CAD build for the part. Positions are in the model's coordinates, mm. A direction names the side the tool comes from. Round coordinates to 2 decimals unless told otherwise and drop trailing zeros. Order: outer loops, then holes, each group sorted by start corner. A loop starts at its lowest first (then second) coordinate and runs counter-clockwise, first axis right, second up. Notation, with made-up numbers: (-35.75, 65.5) -> (20.25, 65.5) arc R11 ccw to (20.25, 77.5) -> close; hole circle Ø5 at (-2.5, 89). An arc over 180 degrees is marked (long way). Answer as CSV lines item,"result". Start each with the question number.
from build123d import *
from build123d.topology import SkipClean

# Parameters (mm, degrees)
SKETCH1_R           = 4
SKETCH1_R_2         = 5.5
BOSS_EXTRUDE1_DEPTH = 2.5
BOSS_EXTRUDE2_START = -5
SKETCH2_R           = 4
BOSS_EXTRUDE2_DEPTH = 5
SKETCH3_R           = 2.25
CUT_EXTRUDE1_DEPTH  = 38.003378224
CUT_EXTRUDE2_DEPTH  = 6
CHAMFER1_SIZE       = 2
FILLET1_R           = 5
BOSS_EXTRUDE3_DEPTH = 10


# Read off the part's stored shape, not the designer's step: Boss-Extrude3
with BuildPart() as part:
    # Sketch1 → Boss-Extrude1 (new, symmetric)
    with BuildSketch(Plane(origin=(0, 0, 0), x_dir=(0, 0, -1), z_dir=(1, 0, 0))):
        with BuildLine():
            Line((-3.149551455, -9.491065569), (15.007926117, -15.51651229))
            ThreePointArc((15.007926117, -15.51651229), (20.188852348, -15.744399678), (24.717514421, -13.217514421))
            Line((24.717514421, -13.217514421), (27.121320344, -10.813708499))
            ThreePointArc((27.121320344, -10.813708499), (27.771638598, -9.840438453), (28, -8.692388155))
            Line((28, -8.692388155), (28, 23))
            Line((28, 23), (18, 23))
            Line((18, 23), (18, 13))
            ThreePointArc((18, 13), (17.121320344, 10.878679656), (15, 10))
            Line((15, 10), (0, 10))
            ThreePointArc((0, 10), (-9.871946507, 1.595202857), (-3.149551455, -9.491065569))
        make_face()
        Circle(SKETCH1_R, mode=Mode.SUBTRACT)
        with Locations((18, -6.5)):
            Circle(SKETCH1_R_2, mode=Mode.SUBTRACT)
    extrude(amount=BOSS_EXTRUDE1_DEPTH, both=True)

    # Sketch2 → Boss-Extrude2 (add)
    with SkipClean():  # the faces are left unmerged after this step: merging them gives an invalid solid
        with BuildSketch(Plane.ZY.offset(-2.5).offset(BOSS_EXTRUDE2_START)):
            with BuildLine():
                Line((0, 10), (-15, 10))
                ThreePointArc((-15, 10), (-17.121320344, 10.878679656), (-18, 13))
                Line((-18, 13), (-18, 23))
                Line((-18, 23), (-28, 23))
                Line((-28, 23), (-28, 9))
                ThreePointArc((-28, 9), (-27.414213562, 7.585786438), (-26, 7))
                Line((-26, 7), (-10.908712115, 7))
                ThreePointArc((-10.908712115, 7), (-9.225461292, 6.08012345), (-9.090593429, 4.166666667))
                ThreePointArc((-9.090593429, 4.166666667), (-9.651431629, 2.617225154), (-9.950203687, 0.996717904))
                ThreePointArc((-9.950203687, 0.996717904), (-7.653907103, -2.763910898), (-7.017714401, -7.124021658))
                ThreePointArc((-7.017714401, -7.124021658), (9.253113438, -3.792082767), (0, 10))
            make_face()
            Circle(SKETCH2_R, mode=Mode.SUBTRACT)
        extrude(amount=BOSS_EXTRUDE2_DEPTH)

    # Sketch3 → Cut-Extrude1 (cut, through all)
    with SkipClean():  # the faces are left unmerged after this step: merging them gives an invalid solid
        with BuildSketch(Plane.XY.offset(-18)):
            with Locations((2.5, 17)):
                Circle(SKETCH3_R)
        extrude(amount=-CUT_EXTRUDE1_DEPTH, mode=Mode.SUBTRACT)

    # Sketch4 → Cut-Extrude2 (cut)
    with SkipClean():  # the faces are left unmerged after this step: merging them gives an invalid solid
        with BuildSketch(Plane(origin=(0, 0, -28), x_dir=(-1, 0, 0), z_dir=(0, 0, -1))):
            Polygon((-6.05, 14.950406544), (-2.5, 12.900813089), (1.05, 14.950406544), (1.05, 19.049593456), (-2.5, 21.099186911), (-6.05, 19.049593456), align=None)
        extrude(amount=-CUT_EXTRUDE2_DEPTH, mode=Mode.SUBTRACT)

    # Chamfer1
    chamfer1_edges = [part.edges().sort_by_distance(p)[0] for p in [
        (-2.5, 23, -23),
        (7.5, 23, -23),
    ]]
    chamfer(chamfer1_edges, length=CHAMFER1_SIZE)

    # Fillet1
    fillet1_edges = [part.edges().sort_by_distance(p)[0] for p in [
        (5, -7.124021658, -7.017714401),
        (5, 0.996717904, -9.950203687),
    ]]
    fillet(fillet1_edges, radius=FILLET1_R)

    # Boss-Extrude3 outline → Boss-Extrude3 (add)
    with SkipClean():  # the faces are left unmerged after this step: merging them gives an invalid solid
        with BuildSketch(Plane(origin=(7.5, 0, 0), x_dir=(0, 0, -1), z_dir=(1, 0, 0))):
            with BuildLine():
                ThreePointArc((-2.463364838, -9.691843668), (0.945667306, -9.955185249), (4.244142914, -9.054681161))
                ThreePointArc((4.244142914, -9.054681161), (6.167964396, -7.465154449), (7.083924127, -5.143796649))
                ThreePointArc((7.083924127, -5.143796649), (7.6539625, -2.763757496), (8.736132305, -0.568663276))
                ThreePointArc((8.736132305, -0.568663276), (9.511605201, 1.757812047), (9.087599302, 4.173192895))
                ThreePointArc((9.087599302, 4.173192895), (7.137011683, 7.00450314), (4.342750079, 9.007803381))
                Line((4.342750079, 9.007803381), (2.44029991, 3.780864498))
                ThreePointArc((2.44029991, 3.780864498), (4.228616794, -1.539090645), (-0.560914668, -4.464904785))
                Line((-0.560914668, -4.464904785), (-2.463364838, -9.691843668))
            make_face()
        extrude(amount=BOSS_EXTRUDE3_DEPTH)


solid = part.part
Item 1: Band-saw the part on D-D, the plane x = 4. Count the separate pieces of the cut face and the enclosed holes in it, and give its area (3 significant figures).
Item 2: Probe line 1 (X direction, y = 17, z = -19.7); line 2 (Z direction, x = 0.25, y = 0); line 3 (X direction, y = 4, z = 7.5). List the from-to ranges inside material, lowest first.
Item 3: Band-saw the part on B-B, the plane z = -14.5. Give the cut face in (x, y).
Item 4: Tool access for faces 5 (the flat face through (0.75, 13.91, -25.04)), 6 (the flat face through (4, 19, -18)), 7 (the flat face through (5, 7, -19)): list every direction of +Z, -Z, +X, -X, +Y, -Y with a clear straight run to the whole face (end or side of a thin tool).
Item 5: Band-saw the part on A-A, the plane y = 17. Give the cut face in (x, z).
Item 6: Band-saw the part on C-C, the plane x = 13. Give the cut face in (y, z).
Item 7: Mould opens along Y. For faces 1 (the flat face through (17.5, -2, -5)), 2 (the flat face through (-1.05, 17, -25)), 3 (the flat face through (4.3, 13.94, -25.04)), 4 (the cylindrical face through (12.43, -7.49, -6.15)) say: released by +Y, released by -Y, zero draft, split by the parting line, or undercut.
Item 8: Pin check, flat tips, straight feed: pin 1 (4 mm diameter, centred on x = 5, z = -20, fed in from -Y); pin 2 (6.5 mm diameter, centred on y = -6.5, z = -18, fed in from +X); pin 3 (1.5 mm diameter, centred on x = 12, y = -10, fed in from -Z); pin 4 (5 mm diameter, centred on x = 3.5, z = -8, fed in from +Y). Stop position of each tip, or through.
Values:
1,separate pieces,"2"
1,enclosed holes,"1"
1,area,"402 mm²"
2,line 1,"-2.5 to 0.25, 4.75 to 7.5"
2,line 2,"-28 to -4, 4 to 10"
2,line 3,"-2.5 to 7.5"
3,outline,"(-2.5, -15.35) -> (2.5, -15.35) -> (2.5, -10.74) -> (-2.5, -10.74) -> close; (-2.5, -2.26) -> (2.5, -2.26) -> (2.5, 7) -> (7.5, 7) -> (7.5, 10) -> (-2.5, 10) -> close"
4,face 5,"-Z"
4,face 6,"+Z, +X, -X, +Y"
4,face 7,"-Z, +X, -Y"
5,outline,"(-2.5, -28) -> (-1.05, -28) -> (-1.05, -22) -> (0.25, -22) -> (0.25, -18) -> (-2.5, -18) -> close; (4.75, -22) -> (6.05, -22) -> (6.05, -28) -> (7.5, -28) -> (7.5, -18) -> (4.75, -18) -> close"
6,outline,"(-9.69, 2.46) arc R10 ccw to (-9.05, -4.24) arc R5 ccw to (-5.14, -7.08) arc R11 cw to (-0.57, -8.74) arc R5 ccw to (4.17, -9.09) arc R10 ccw to (9.01, -4.34) -> (3.78, -2.44) arc R4.5 cw to (-4.46, 0.56) -> close"
7,face 1,"zero draft"
7,face 2,"undercut"
7,face 3,"undercut"
7,face 4,"released by -Y"
8,pin 1,"y = 7"
8,pin 2,"through"
8,pin 3,"z = -3.8"
8,pin 4,"y = 10"
